Read the model definition and answer for the solid it produces. Units are mm, in the model's axes. Face numbers are marked on the shaded views. A direction names the side the tool comes from. Give positions to 0.01 mm unless a question says otherwise; leave off trailing zeros. Loops run counter-clockwise (first coordinate to the right, second up) from the corner with the lowest first, then second, coordinate; pieces in that order, holes last.
(1) Find section C-C, the plane z = 5. Write down the section's boundary in (x, y).
(2) Find section D-D, the plane y = 6.75. Write down the section's boundary in (x, z), then the cut area to 3 significant figures.
(3) Find section B-B, the plane x = -8. Write down the section's boundary in (y, z), then the cut area to 3 significant figures.
(4) Determine the mould class of the marked faces 6, 7 and 8 for opening direction Y: pulls with the +Y half, pulls with the -Y half, needs draft (parallel to the pull), parting line crosses it, or undercut.
(5) Find section A-A, the plane z = -3. Write down the section's boundary in (x, y).
(6) Which of the six approach directions +Z, -Z, +X, -X, +Y, -Y give full straight-line access (tool end or side, diameter ignored) to the marked faces 1, 2, 3, 4 and 5?
(7) Straight lines are drawn through the part: probe 1 along X at (y, z) = (5.5, 3.75); probe 2 along Z at (x, y) = (-6.25, 7.75); probe 3 along Y at (x, z) = (0, -4.25). For each, find the intervals that lie inside material, in ascending order.
(8) Each of these flat-tipped pins is pushed along its axis until it touches: P1, Ø5, axis at x = -3, z = -10, coming from the +Y side; P2, Ø0.6, axis at x = -2.5, z = -0.5, coming from the -Y side; P3, Ø3, axis at x = 5.5, z = -11, coming from the -Y side. Where does it stop, or does it pass through?
```python
from build123d import *

# Parameters (mm, degrees)
F0_R            = 5.85
F1_DEPTH        = 14
F2_W            = 19
F2_H            = 17
F3_DEPTH        = 4
F4_W            = 19
F4_H            = 2.3
F5_DEPTH        = 1
F7_DEPTH        = 1.5
F7_COPIES_COUNT = 4
F9_DEPTH        = 14.5
F10_R           = 2.5
F11_DEPTH       = 15
F12_R           = 2
F13_T1_DEPTH    = 19
F13_T6_ANGLE    = 84.7754573572
F13_T12_ANGLE   = 84.7754573572
F13_T18_ANGLE   = 84.7754573572
F13_T24_ANGLE   = 84.7754573572
F13_T30_ANGLE   = 96.86145484
F13_T36_ANGLE   = 96.86145484
F13_T43_ANGLE   = 96.86145484
F13_T47_DEPTH   = 20.497881522
F13_T54_ANGLE   = 96.86145484
F13_T58_DEPTH   = 20.497881522


# Not quite as in the source:
# - a fillet or chamfer that OpenCascade refuses, or shapes differently, is made with other operations: its cross-section is extruded or revolved along the edge and cut away or added
# - a pattern or mirror of a feature is missing from the dataset's text; its kind, count and spacing are read off the source's solid


with BuildPart() as f1:
    # F0 (on Top) → F1 (new body)
    with BuildSketch(Plane.XY):
        Circle(F0_R)
    extrude(amount=-F1_DEPTH)

    # F2 (on Top) → F3 (join)
    with BuildSketch(Plane.XY):
        with Locations((0, 2.65)):
            Rectangle(F2_W, F2_H)
    extrude(amount=F3_DEPTH)

    # F4 (on Top) → F5 (join)
    with BuildSketch(Plane.XY):
        with Locations((0, 10)):
            Rectangle(F4_W, F4_H)
    extrude(amount=-F5_DEPTH)

    # F6 (on Front) → F7 (join, symmetric)
    with BuildSketch(Plane.XZ):
        Polygon((6, -10), (6.3, 0), (5, 0), (5, -10), align=None)
    f7 = extrude(amount=F7_DEPTH, both=True)

    # F7_copies: F7 ×4 about axis
    f7_copies_axis = Axis((0, 0, 0), (0, 0, 1))
    for i in range(1, F7_COPIES_COUNT):
        add(f7.rotate(f7_copies_axis, i * 360 / F7_COPIES_COUNT))

    # F8 (on Right) → F9 (join, symmetric)
    with BuildSketch(Plane.YZ):
        with BuildLine():
            Line((12.15, 4), (8.2770166538, 4))
            ThreePointArc((8.2770166538, 4), (16.0871501864, 4.2937079857), (8.8661178186, 7.2838821814))
            Line((8.8661178186, 7.2838821814), (12.15, 4))
        make_face()
    extrude(amount=F9_DEPTH, both=True)

    # F10 (on Top) → F11 (cut, symmetric)
    with BuildSketch(Plane.XY):
        Circle(F10_R)
    extrude(amount=F11_DEPTH, both=True, mode=Mode.SUBTRACT)

    # F12
    f12_edges = [f1.edges().sort_by_distance(p)[0] for p in [
        (-9.5, -5.85, 2),
        (9.5, -5.85, 2),
        (-2.5, 0, -14),
        (-2.5, 0, 4),
    ]]
    fillet(f12_edges, radius=F12_R)

    # F13: fillet of radius 0.5 on 9 edges, made by hand

    # F13_s2 → F13_t1 (join)
    with BuildSketch(Plane.YZ.offset(-9.5)):
        with BuildLine():
            ThreePointArc((8.35, 0), (8.7035533906, -0.1464466094), (8.85, -0.5))
            Line((8.85, -0.5), (8.85, 0))
            Line((8.85, 0), (8.35, 0))
        make_face()
        with BuildLine():
            ThreePointArc((11.7055555556, 1.02476804), (11.3166666667, 0.9005420413), (11.15, 0.527864045))
            Line((11.15, 0.527864045), (11.15, 1.1270166538))
            ThreePointArc((11.15, 1.1270166538), (11.4259705579, 1.0660730349), (11.7055555556, 1.02476804))
        make_face()
    extrude(amount=F13_T1_DEPTH)


with BuildPart() as f13_tool4:
    # F13_s5 → F13_t6 (revolve)
    with BuildSketch(Plane(origin=(0, 0, 0), x_dir=(0, 0, 1), z_dir=(-0.9989608313, -0.0455769416, 0))):
        with BuildLine():
            ThreePointArc((0, -6.35), (-0.1464466094, -5.9964466094), (-0.5, -5.85))
            Line((-0.5, -5.85), (0, -5.85))
            Line((0, -5.85), (0, -6.35))
        make_face()
    revolve(axis=Axis((0, 0, 0), (0, 0, 1)), revolution_arc=F13_T6_ANGLE)

    split(bisect_by=Plane(origin=(6.2943350984, 0, -0.188830053), x_dir=(0, 1, 0), z_dir=(-0.9995503035, 0, 0.0299865091)), keep=Keep.TOP)

    split(bisect_by=Plane(origin=(0, -6.2943350984, -0.188830053), x_dir=(1, 0, 0), z_dir=(0, 0.9995503035, 0.0299865091)), keep=Keep.TOP)


with BuildPart() as f1_1:
    add(f1.part)

    # F13_t3: union F13_tool4
    add(f13_tool4.part)


with BuildPart() as f13_tool10:
    # F13_s11 → F13_t12 (revolve)
    with BuildSketch(Plane(origin=(0, 0, 0), x_dir=(0, 0, 1), z_dir=(0.0455769416, -0.9989608313, 0))):
        with BuildLine():
            ThreePointArc((0, -6.35), (-0.1464466094, -5.9964466094), (-0.5, -5.85))
            Line((-0.5, -5.85), (0, -5.85))
            Line((0, -5.85), (0, -6.35))
        make_face()
    revolve(axis=Axis((0, 0, 0), (0, 0, 1)), revolution_arc=F13_T12_ANGLE)

    split(bisect_by=Plane.XZ.offset(-1.5), keep=Keep.BOTTOM)

    split(bisect_by=Plane(origin=(0, 6.2943350984, -0.188830053), x_dir=(1, 0, 0), z_dir=(0, -0.9995503035, 0.0299865091)), keep=Keep.TOP)


with BuildPart() as f1_2:
    add(f1_1.part)

    # F13_t9: union F13_tool10
    add(f13_tool10.part)


with BuildPart() as f13_tool16:
    # F13_s17 → F13_t18 (revolve)
    with BuildSketch(Plane(origin=(0, 0, 0), x_dir=(0, 0, 1), z_dir=(0.9989608313, 0.0455769416, 0))):
        with BuildLine():
            ThreePointArc((0, -6.35), (-0.1464466094, -5.9964466094), (-0.5, -5.85))
            Line((-0.5, -5.85), (0, -5.85))
            Line((0, -5.85), (0, -6.35))
        make_face()
    revolve(axis=Axis((0, 0, 0), (0, 0, 1)), revolution_arc=F13_T18_ANGLE)

    split(bisect_by=Plane.XZ.offset(-1.5), keep=Keep.BOTTOM)

    split(bisect_by=Plane.YZ.offset(-1.5), keep=Keep.BOTTOM)


with BuildPart() as f1_3:
    add(f1_2.part)

    # F13_t15: union F13_tool16
    add(f13_tool16.part)


with BuildPart() as f13_tool22:
    # F13_s23 → F13_t24 (revolve)
    with BuildSketch(Plane(origin=(0, 0, 0), x_dir=(0, 0, 1), z_dir=(-0.0455769416, 0.9989608313, 0))):
        with BuildLine():
            ThreePointArc((0, -6.35), (-0.1464466094, -5.9964466094), (-0.5, -5.85))
            Line((-0.5, -5.85), (0, -5.85))
            Line((0, -5.85), (0, -6.35))
        make_face()
    revolve(axis=Axis((0, 0, 0), (0, 0, 1)), revolution_arc=F13_T24_ANGLE)

    split(bisect_by=Plane(origin=(-6.2943350984, 0, -0.188830053), x_dir=(0, 1, 0), z_dir=(0.9995503035, 0, 0.0299865091)), keep=Keep.TOP)

    split(bisect_by=Plane(origin=(0, -6.2943350984, -0.188830053), x_dir=(1, 0, 0), z_dir=(0, 0.9995503035, 0.0299865091)), keep=Keep.TOP)


with BuildPart() as f1_4:
    add(f1_3.part)

    # F13_t21: union F13_tool22
    add(f13_tool22.part)


with BuildPart() as f13_tool28:
    # F13_s29 → F13_t30 (revolve)
    with BuildSketch(Plane(origin=(0, 0.3421818863, 5.7078686812), x_dir=(1, 0, 0), z_dir=(0, 0.0598417157, 0.9982078787))):
        with BuildLine():
            ThreePointArc((-9.5, 7.3290171475), (-9.6464466094, 7.6825705381), (-10, 7.8290171475))
            Line((-10, 7.8290171475), (-9.5, 7.8290171475))
            Line((-9.5, 7.8290171475), (-9.5, 7.3290171475))
        make_face()
    revolve(axis=Axis((-9.5, 12.15, 5), (1, 0, 0)), revolution_arc=F13_T30_ANGLE)

    split(bisect_by=Plane.XY.offset(4), keep=Keep.BOTTOM)

    split(bisect_by=Plane.XZ.offset(-11.15), keep=Keep.TOP)


with BuildPart() as f1_5:
    add(f1_4.part)

    # F13_t27: union F13_tool28
    add(f13_tool28.part)


with BuildPart() as f13_tool34:
    # F13_s35 → F13_t36 (revolve)
    with BuildSketch(Plane(origin=(0, 0.3421818863, 5.7078686812), x_dir=(1, 0, 0), z_dir=(0, 0.0598417157, 0.9982078787))):
        with BuildLine():
            ThreePointArc((9.5, 7.3290171475), (9.6464466094, 7.6825705381), (10, 7.8290171475))
            Line((10, 7.8290171475), (9.5, 7.8290171475))
            Line((9.5, 7.8290171475), (9.5, 7.3290171475))
        make_face()
    revolve(axis=Axis((9.5, 12.15, 5), (1, 0, 0)), revolution_arc=F13_T36_ANGLE)

    split(bisect_by=Plane.XY.offset(4), keep=Keep.BOTTOM)

    split(bisect_by=Plane.XZ.offset(-11.15), keep=Keep.TOP)


with BuildPart() as f1_6:
    add(f1_5.part)

    # F13_t33: union F13_tool34
    add(f13_tool34.part)


with BuildPart() as f13_tool41:
    # F13_s42 → F13_t43 (revolve)
    with BuildSketch(Plane(origin=(0, 0.3421818863, 5.7078686812), x_dir=(1, 0, 0), z_dir=(0, 0.0598417157, 0.9982078787))):
        with BuildLine():
            ThreePointArc((-9.5, 7.3290171475), (-9.6464466094, 7.6825705381), (-10, 7.8290171475))
            Line((-10, 7.8290171475), (-9.5, 7.8290171475))
            Line((-9.5, 7.8290171475), (-9.5, 7.3290171475))
        make_face()
    revolve(axis=Axis((-9.5, 12.15, 5), (1, 0, 0)), revolution_arc=F13_T43_ANGLE)

    split(bisect_by=Plane.XZ.offset(-11.15), keep=Keep.BOTTOM)


with BuildPart() as f13_tool45:
    # F13_s46 → F13_t47 (new body)
    with BuildSketch(Plane.YZ.offset(-10.997881522)):
        with BuildLine():
            ThreePointArc((11.7055555556, 1.02476804), (11.3166666667, 0.9005420413), (11.15, 0.527864045))
            Line((11.15, 0.527864045), (11.15, 1.1270166538))
            ThreePointArc((11.15, 1.1270166538), (11.4259705579, 1.0660730349), (11.7055555556, 1.02476804))
        make_face()
    extrude(amount=F13_T47_DEPTH)

    split(bisect_by=Plane.YZ.offset(-9.5), keep=Keep.BOTTOM)


with BuildPart() as f13_tool41_1:
    add(f13_tool41.part)

    # F13_t49: intersect F13_tool45
    add(f13_tool45.part, mode=Mode.INTERSECT)


with BuildPart() as f1_7:
    add(f1_6.part)

    # F13_t39: union F13_tool41
    add(f13_tool41_1.part)


with BuildPart() as f13_tool52:
    # F13_s53 → F13_t54 (revolve)
    with BuildSketch(Plane(origin=(0, 0.3421818863, 5.7078686812), x_dir=(1, 0, 0), z_dir=(0, 0.0598417157, 0.9982078787))):
        with BuildLine():
            ThreePointArc((9.5, 7.3290171475), (9.6464466094, 7.6825705381), (10, 7.8290171475))
            Line((10, 7.8290171475), (9.5, 7.8290171475))
            Line((9.5, 7.8290171475), (9.5, 7.3290171475))
        make_face()
    revolve(axis=Axis((9.5, 12.15, 5), (1, 0, 0)), revolution_arc=F13_T54_ANGLE)

    split(bisect_by=Plane.XZ.offset(-11.15), keep=Keep.BOTTOM)


with BuildPart() as f13_tool56:
    # F13_s57 → F13_t58 (new body)
    with BuildSketch(Plane.YZ.offset(-9.5)):
        with BuildLine():
            ThreePointArc((11.7055555556, 1.02476804), (11.3166666667, 0.9005420413), (11.15, 0.527864045))
            Line((11.15, 0.527864045), (11.15, 1.1270166538))
            ThreePointArc((11.15, 1.1270166538), (11.4259705579, 1.0660730349), (11.7055555556, 1.02476804))
        make_face()
    extrude(amount=F13_T58_DEPTH)

    split(bisect_by=Plane.YZ.offset(9.5), keep=Keep.TOP)


with BuildPart() as f13_tool52_1:
    add(f13_tool52.part)

    # F13_t60: intersect F13_tool56
    add(f13_tool56.part, mode=Mode.INTERSECT)


with BuildPart() as f1_8:
    add(f1_7.part)

    # F13_t50: union F13_tool52
    add(f13_tool52_1.part)

    # F13_s61 → F13_t62 (revolve, cut)
    with BuildSketch(Plane.XZ):
        with BuildLine():
            ThreePointArc((5.85, -13.5), (5.7035533906, -13.8535533906), (5.35, -14))
            Line((5.35, -14), (5.85, -14))
            Line((5.85, -14), (5.85, -13.5))
        make_face()
    revolve(axis=Axis((0, 0, -14), (0, 0, 1)), mode=Mode.SUBTRACT)


solid = f1_8.part
```
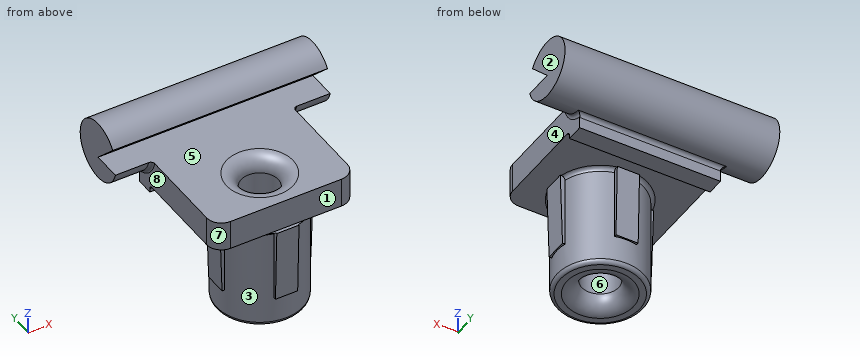
Entries:
1. outline: (-14.5, 11.15) - (14.5, 11.15) - (14.5, 16.15) - (-14.5, 16.15) - close
2. outline: (-9.5, 0) - (9.5, 0) - (9.5, 4) - (-9.5, 4) - close
2. area: 76.0 mm2
3. outline: (-5.79, 0) - (8.35, 0) arc R0.5 cw to (8.85, -0.5) - (8.85, -1) - (11.15, -1) - (11.15, 0.53) arc R0.5 cw to (11.71, 1.02) arc R4 ccw (long way) to (8.87, 7.28) - (12.15, 4) - (-5.79, 4) - close
3. area: 108 mm2
4. face 6: undercut
4. face 7: pulls with the -Y half
4. face 8: needs draft
5. outline: (-6.21, -1.5) - (-5.65, -1.5) arc R5.85 ccw to (-1.5, -5.65) - (-1.5, -6.21) - (1.5, -6.21) - (1.5, -5.65) arc R5.85 ccw to (5.65, -1.5) - (6.21, -1.5) - (6.21, 1.5) - (5.65, 1.5) arc R5.85 ccw to (1.5, 5.65) - (1.5, 6.21) - (-1.5, 6.21) - (-1.5, 5.65) arc R5.85 ccw to (-5.65, 1.5) - (-6.21, 1.5) - close; hole circle Ø5 at (0, 0)
6. face 1: +Z, +X, -X, -Y
6. face 2: +Z, -Z, +X, +Y, -Y
6. face 3: -Z
6. face 4: -Z, +X, -Y
6. face 5: +X, -X, -Y
7. probe 1: x = -9.5 to 9.5
7. probe 2: z = 0 to 4
7. probe 3: y = -6.17 to -2.5, 2.5 to 6.17
8. P1: stops at y = 6.06
8. P2: stops at y = -5.44
8. P3: stops at y = -4.27
